from build123d import *

# Parameters (mm, degrees)
SKETCH2_W                    = 254
SKETCH2_H                    = 254
BOSS_EXTRUDE1_DEPTH          = 1.00076
SKETCH3_W                    = 69.85
SKETCH3_H                    = 25.4
CUT_EXTRUDE1_DEPTH           = 1
CUT_EXTRUDE1_DEPTH_BACK      = 2.00076
CUT_EXTRUDE2_DEPTH           = 1
CUT_EXTRUDE2_DEPTH_BACK      = 2.00076
SKETCH5_R                    = 2.150000018
CUT_EXTRUDE3_DEPTH           = 1
CUT_EXTRUDE3_DEPTH_BACK      = 2.00076
SKETCH6_R                    = 2.099999991
CUT_EXTRUDE4_DEPTH           = 1
CUT_EXTRUDE4_DEPTH_BACK      = 2.00076
SKETCH7_W                    = 95.25
SKETCH7_H                    = 95.25
CUT_EXTRUDE5_DEPTH           = 1
CUT_EXTRUDE5_DEPTH_BACK      = 2.00076
CUT_EXTRUDE6_DEPTH           = 1
CUT_EXTRUDE6_DEPTH_BACK      = 2.00076
BOSS_EXTRUDE4_DEPTH          = 1.00076
SKETCH18_W                   = 12.7
SKETCH18_H                   = 1.27
CUT_EXTRUDE_THIN4_DEPTH      = 1
CUT_EXTRUDE_THIN4_DEPTH_BACK = 2.00076
CUT_EXTRUDE7_DEPTH           = 1
CUT_EXTRUDE7_DEPTH_BACK      = 2.00076
SKETCH10_W                   = 9.525
SKETCH10_H                   = 60.6472
SKETCH10_W_2                 = 95.25
SKETCH10_H_2                 = 9.525
BOSS_EXTRUDE2_DEPTH          = 1.00076
SKETCH14_R                   = 2.200000045
BOSS_EXTRUDE3_DEPTH          = 1.00076
SKETCH15_W                   = 1.27
SKETCH15_H                   = 6.35
CUT_EXTRUDE_THIN3_DEPTH      = 1
CUT_EXTRUDE_THIN3_DEPTH_BACK = 2.00076
SKETCH19_R                   = 1.5875
CUT_EXTRUDE8_DEPTH           = 1
CUT_EXTRUDE8_DEPTH_BACK      = 2.00076
SKETCH20_W                   = 1.27
SKETCH20_H                   = 1.27
SKETCH20_W_2                 = 6.35
CUT_EXTRUDE12_DEPTH          = 1
CUT_EXTRUDE12_DEPTH_BACK     = 2.00076


with BuildPart() as part:
    # Sketch2 → Boss-Extrude1 (new body)
    with BuildSketch(Plane(origin=(0, 0, 0), x_dir=(1, 0, 0), z_dir=(0, 1, 0))):
        Rectangle(SKETCH2_W, SKETCH2_H)
    extrude(amount=BOSS_EXTRUDE1_DEPTH)

    # Sketch3 → Cut-Extrude1 (cut, two sides)
    with BuildSketch(Plane(origin=(0, 1.00076, 0), x_dir=(1, 0, 0), z_dir=(0, 1, 0))) as cut_extrude1_sk:
        with Locations((92.075, 34.552)):
            Rectangle(SKETCH3_W, SKETCH3_H)
    extrude(amount=CUT_EXTRUDE1_DEPTH, mode=Mode.SUBTRACT)
    extrude(cut_extrude1_sk.sketch, amount=-CUT_EXTRUDE1_DEPTH_BACK, mode=Mode.SUBTRACT)

    # Sketch4 → Cut-Extrude2 (cut, two sides)
    with BuildSketch(Plane(origin=(0, 1.00076, 0), x_dir=(1, 0, 0), z_dir=(0, 1, 0))) as cut_extrude2_sk:
        with BuildLine():
            Line((127, -127), (127, 21.852))
            Line((127, 21.852), (122.640015225, 21.852))
            ThreePointArc((122.640015225, 21.852), (94.909945844, -51.086516198), (112.96892893, -127))
            Line((112.96892893, -127), (127, -127))
        make_face()
    extrude(amount=CUT_EXTRUDE2_DEPTH, mode=Mode.SUBTRACT)
    extrude(cut_extrude2_sk.sketch, amount=-CUT_EXTRUDE2_DEPTH_BACK, mode=Mode.SUBTRACT)

    # Sketch5 → Cut-Extrude3 (cut, two sides)
    with BuildSketch(Plane(origin=(0, 1.00076, 0), x_dir=(1, 0, 0), z_dir=(0, 1, 0))) as cut_extrude3_sk:
        with Locations((69.85, -123.19)):
            Circle(SKETCH5_R)
        with Locations((101.802396213, -123.19)):
            Circle(SKETCH5_R)
        with Locations((66.977000031, 17.859999967)):
            Circle(SKETCH5_R)
        with Locations((115.577000113, 17.859999967)):
            Circle(SKETCH5_R)
    extrude(amount=CUT_EXTRUDE3_DEPTH, mode=Mode.SUBTRACT)
    extrude(cut_extrude3_sk.sketch, amount=-CUT_EXTRUDE3_DEPTH_BACK, mode=Mode.SUBTRACT)

    # Sketch6 → Cut-Extrude4 (cut, two sides)
    with BuildSketch(Plane(origin=(0, 1.00076, 0), x_dir=(1, 0, 0), z_dir=(0, 1, 0))) as cut_extrude4_sk:
        with Locations((66.977000031, 27.860000033)):
            Circle(SKETCH6_R)
        with Locations((66.977000031, 17.859999967)):
            Circle(SKETCH6_R)
        with Locations((115.577000113, 27.860000033)):
            Circle(SKETCH6_R)
        with Locations((115.577000113, 17.859999967)):
            Circle(SKETCH6_R)
        Polygon((70.700000078, 22.36), (70.700000078, 12.733000061), (111.854000066, 12.733000061), (111.854000066, 22.36), (118.458000066, 22.36), (118.458000066, 23.36), (111.854000066, 23.36), (111.854000066, 32.986999939), (70.700000078, 32.986999939), (70.700000078, 23.36), (64.096000078, 23.36), (64.096000078, 22.36), align=None)
    extrude(amount=CUT_EXTRUDE4_DEPTH, mode=Mode.SUBTRACT)
    extrude(cut_extrude4_sk.sketch, amount=-CUT_EXTRUDE4_DEPTH_BACK, mode=Mode.SUBTRACT)

    # Sketch7 → Cut-Extrude5 (cut, two sides)
    with BuildSketch(Plane(origin=(0, 1.00076, 0), x_dir=(1, 0, 0), z_dir=(0, 1, 0))) as cut_extrude5_sk:
        with Locations((12.1158, 50.1142)):
            Rectangle(SKETCH7_W, SKETCH7_H)
    extrude(amount=CUT_EXTRUDE5_DEPTH, mode=Mode.SUBTRACT)
    extrude(cut_extrude5_sk.sketch, amount=-CUT_EXTRUDE5_DEPTH_BACK, mode=Mode.SUBTRACT)

    # Sketch8 → Cut-Extrude6 (cut, two sides)
    with BuildSketch(Plane(origin=(0, 1.00076, 0), x_dir=(1, 0, 0), z_dir=(0, 1, 0))) as cut_extrude6_sk:
        Polygon((127, 47.252), (127, 127), (-127, 127), (-127, -127), (-35.5092, -127), (-35.5092, 47.252), align=None)
    extrude(amount=CUT_EXTRUDE6_DEPTH, mode=Mode.SUBTRACT)
    extrude(cut_extrude6_sk.sketch, amount=-CUT_EXTRUDE6_DEPTH_BACK, mode=Mode.SUBTRACT)

    # Sketch17 → Boss-Extrude4 (add)
    with BuildSketch(Plane(origin=(0, 1.00076, 0), x_dir=(1, 0, 0), z_dir=(0, 1, 0))):
        Polygon((59.7408, 2.4892), (47.0408, 2.4892), (47.0408, 97.7392), (59.7408, 97.7392), (154.9908, 97.7392), (154.9908, 85.0392), (59.7408, 85.0392), align=None)
    extrude(amount=-BOSS_EXTRUDE4_DEPTH)

    # Sketch18 → Cut-Extrude-Thin4 (cut, two sides)
    with BuildSketch(Plane(origin=(0, 1.00076, 0), x_dir=(1, 0, 0), z_dir=(0, 1, 0))) as cut_extrude_thin4_sk:
        with Locations((53.3908, 3.1242)):
            Rectangle(SKETCH18_W, SKETCH18_H)
    extrude(amount=CUT_EXTRUDE_THIN4_DEPTH, mode=Mode.SUBTRACT)
    extrude(cut_extrude_thin4_sk.sketch, amount=-CUT_EXTRUDE_THIN4_DEPTH_BACK, mode=Mode.SUBTRACT)

    # Sketch9 → Cut-Extrude7 (cut, two sides)
    with BuildSketch(Plane(origin=(0, 1.00076, 0), x_dir=(1, 0, 0), z_dir=(0, 1, 0))) as cut_extrude7_sk:
        Polygon((-35.5092, -55.113847322), (36.376952678, -127), (-35.5092, -127), align=None)
    extrude(amount=CUT_EXTRUDE7_DEPTH, mode=Mode.SUBTRACT)
    extrude(cut_extrude7_sk.sketch, amount=-CUT_EXTRUDE7_DEPTH_BACK, mode=Mode.SUBTRACT)

    # Sketch10 → Boss-Extrude2 (add)
    with BuildSketch(Plane(origin=(0, 1.00076, 0), x_dir=(1, 0, 0), z_dir=(0, 1, 0))):
        with Locations((64.5033, 53.4456)):
            Rectangle(SKETCH10_W, SKETCH10_H)
        with Locations((107.3658, 102.5017)):
            Rectangle(SKETCH10_W_2, SKETCH10_H_2)
    extrude(amount=-BOSS_EXTRUDE2_DEPTH)

    # Sketch14 → Boss-Extrude3 (add)
    with BuildSketch(Plane(origin=(0, 1.00076, 0), x_dir=(1, 0, 0), z_dir=(0, 1, 0))):
        with BuildLine():
            Line((-61.511199939, -50.699323655), (-61.511199939, -9.545323667))
            Line((-61.511199939, -9.545323667), (-51.8842, -9.545323667))
            Line((-51.8842, -9.545323667), (-51.8842, -2.941323667))
            Line((-51.8842, -2.941323667), (-50.8842, -2.941323667))
            Line((-50.8842, -2.941323667), (-50.8842, -5.1308))
            Line((-50.8842, -5.1308), (-48.472691116, -5.1308))
            ThreePointArc((-48.472691116, -5.1308), (-46.384199967, -3.622323575), (-44.295708818, -5.1308))
            Line((-44.295708818, -5.1308), (-35.5092, -5.1308))
            Line((-35.5092, -5.1308), (-35.5092, 2.4892))
            Line((-35.5092, 2.4892), (-67.2592, 2.4892))
            Line((-67.2592, 2.4892), (-67.2592, -73.66))
            Line((-67.2592, -73.66), (-16.963047322, -73.66))
            Line((-16.963047322, -73.66), (-35.5092, -55.113847322))
            Line((-35.5092, -55.113847322), (-44.295708818, -55.113847322))
            ThreePointArc((-44.295708818, -55.113847322), (-46.384199967, -56.622323747), (-48.472691116, -55.113847322))
            Line((-48.472691116, -55.113847322), (-50.8842, -55.113847322))
            Line((-50.8842, -55.113847322), (-50.8842, -57.303323655))
            Line((-50.8842, -57.303323655), (-51.8842, -57.303323655))
            Line((-51.8842, -57.303323655), (-51.8842, -50.699323655))
            Line((-51.8842, -50.699323655), (-61.511199939, -50.699323655))
        make_face()
        with Locations((-56.384200033, -54.422323702)):
            Circle(SKETCH14_R, mode=Mode.SUBTRACT)
        with Locations((-56.384200033, -5.82232362)):
            Circle(SKETCH14_R, mode=Mode.SUBTRACT)
    extrude(amount=-BOSS_EXTRUDE3_DEPTH)

    # Sketch15 → Cut-Extrude-Thin3 (cut, two sides)
    with BuildSketch(Plane(origin=(0, 1.00076, 0), x_dir=(1, 0, 0), z_dir=(0, 1, 0))) as cut_extrude_thin3_sk:
        with Locations((-17.598047322, -70.485)):
            Rectangle(SKETCH15_W, SKETCH15_H)
    extrude(amount=CUT_EXTRUDE_THIN3_DEPTH, mode=Mode.SUBTRACT)
    extrude(cut_extrude_thin3_sk.sketch, amount=-CUT_EXTRUDE_THIN3_DEPTH_BACK, mode=Mode.SUBTRACT)

    # Sketch19 → Cut-Extrude8 (cut, two sides)
    with BuildSketch(Plane(origin=(0, 1.00076, 0), x_dir=(1, 0, 0), z_dir=(0, 1, 0))) as cut_extrude8_sk:
        with Locations((56.5658, -0.6858)):
            Circle(SKETCH19_R)
        with Locations((-32.3342, -0.6858)):
            Circle(SKETCH19_R)
        with Locations((151.8158, 88.2142)):
            Circle(SKETCH19_R)
        with Locations((62.9158, 88.2142)):
            Circle(SKETCH19_R)
    extrude(amount=CUT_EXTRUDE8_DEPTH, mode=Mode.SUBTRACT)
    extrude(cut_extrude8_sk.sketch, amount=-CUT_EXTRUDE8_DEPTH_BACK, mode=Mode.SUBTRACT)

    # Sketch20 → Cut-Extrude12 (cut, two sides)
    with BuildSketch(Plane(origin=(0, 1.00076, 0), x_dir=(1, 0, 0), z_dir=(0, 1, 0))) as cut_extrude12_sk:
        with Locations((59.1058, 84.4042)):
            Rectangle(SKETCH20_W, SKETCH20_H)
        Polygon((59.7408, 91.3892), (66.0908, 91.3892), (66.0908, 92.6592), (58.4708, 92.6592), (58.4708, 85.0392), (59.7408, 85.0392), align=None)
        with Locations((60.3758, 3.1242)):
            Rectangle(SKETCH20_W, SKETCH20_H)
        Polygon((59.7408, -3.8608), (53.3908, -3.8608), (53.3908, -5.1308), (61.0108, -5.1308), (61.0108, 2.4892), (59.7408, 2.4892), align=None)
        Polygon((-29.1592, -3.8608), (-29.1592, -5.1308), (-36.7792, -5.1308), (-36.7792, 2.4892), (-35.5092, 2.4892), (-35.5092, -3.8608), align=None)
        with Locations((151.8158, 92.0242)):
            Rectangle(SKETCH20_W_2, SKETCH20_H)
    extrude(amount=CUT_EXTRUDE12_DEPTH, mode=Mode.SUBTRACT)
    extrude(cut_extrude12_sk.sketch, amount=-CUT_EXTRUDE12_DEPTH_BACK, mode=Mode.SUBTRACT)


solid = part.part
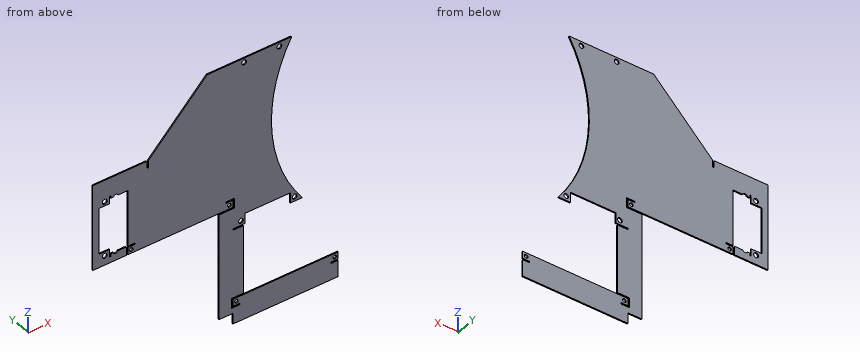
Work out the finished part from the listing and answer in its coordinate system (mm). Give positions to 0.01 mm unless a question says otherwise; leave off trailing zeros. Write each loop counter-clockwise with the first axis right and the second up, starting at its lowest first coordinate (ties: lowest second). Pieces come first, ordered by that corner, then holes. Notation, with made-up numbers: M -30.5,-9 L -23.5,-9 A33 cw -23.5,29 Z; hole C -16.75,38 d11. An arc over 180 degrees is marked long. Answer as CSV lines item,"result".
Q1. Find the intervals of material crossed by probe 1 along Z at (x, y) = (134, 0.15); probe 2 along X at (y, z) = (0.15, 50); probe 3 along X at (y, z) = (0.15, 72), in increasing order. Write a range as [from, to].
A:
probe 1,"z = [-107.26, -85.04]"
probe 2,"x = [-67.26, -61.51], [-35.51, 94.99]"
probe 3,"x = [-67.26, -18.23], [-16.96, 95.2]"
Q2. A cutting plane is placed at A-A on x = 87.5. Write down the section's boundary in (y, z).
A:
outline,"M 0,-107.26 L 1,-107.26 L 1,-85.04 L 0,-85.04 Z; M 0,-12.73 L 1,-12.73 L 1,127 L 0,127 Z"
Q3. Given P1, Ø3.5, axis at x = 115.577, z = -17.86, coming from the +Y side; P2, Ø0.5, axis at x = 4.5, y = 0.5, coming from the -Z side; P3, Ø0.5, axis at x = 151, y = 0.5, coming from the +Z side, each flat-ended and moving along its own axis, determine where each tip first touches the part or whether it passes through.
A:
P1,"passes through"
P2,"stops at z = -2.49"
P3,"stops at z = -85.04"
Q4. A cutting plane is placed at C-C on x = -21. Write down the section's boundary in (y, z).
A:
outline,"M 0,-2.49 L 1,-2.49 L 1,73.66 L 0,73.66 Z"
Q5. A cutting plane is placed at B-B on z = 27. Write down the section's boundary in (x, y), plus the area to 3 significant figures.
A:
outline,"M -67.26,0 L -61.51,0 L -61.51,1 L -67.26,1 Z; M -35.51,0 L 98.72,0 L 98.72,1 L -35.51,1 Z"
area,"140 mm²"
Q6. A cutting plane is placed at D-D on y = 0.65. Count the separate pieces of the cut face and the enclosed holes in it, plus the area to 3 significant figures.
A:
separate pieces,"1"
enclosed holes,"10"
area,"20,800 mm²"
